```python
from build123d import *

# Parameters (mm, degrees)
SKETCH1_W          = 304.8
SKETCH1_H          = 142.24
EXTRUDE1_DEPTH     = 2.032
SKETCH3_R          = 1.5875
CUT_EXTRUDE1_DEPTH = 252.699806613
SKETCH4_R          = 4.191
SKETCH4_R_2        = 1.5875
SKETCH4_R_3        = 5.842
SKETCH4_W          = 80.01
SKETCH4_H          = 44.958
SKETCH4_W_2        = 29.972
SKETCH4_H_2        = 29.972
EXTRUDE2_DEPTH     = 252.699806613


with BuildPart() as part:
    # Sketch1 → Extrude1 (new body)
    with BuildSketch(Plane.XY):
        with Locations((55.245, 71.12)):
            Rectangle(SKETCH1_W, SKETCH1_H)
    extrude(amount=EXTRUDE1_DEPTH)

    # Sketch3 → Cut-Extrude1 (cut, through all)
    with BuildSketch(Plane.XY.offset(2.032)):
        with Locations((-90.805, 135.89)):
            Circle(SKETCH3_R)
        with Locations((-90.805, 6.35)):
            Circle(SKETCH3_R)
        with Locations((6.35, 135.89)):
            Circle(SKETCH3_R)
        with Locations((6.35, 6.35)):
            Circle(SKETCH3_R)
        with Locations(Location((104.14, 6.35, 0), (0, 0, 180))):
            Circle(SKETCH3_R)
        with Locations(Location((104.14, 135.89, 0), (0, 0, 180))):
            Circle(SKETCH3_R)
        with Locations(Location((201.295, 6.35, 0), (0, 0, 180))):
            Circle(SKETCH3_R)
        with Locations(Location((201.295, 135.89, 0), (0, 0, 180))):
            Circle(SKETCH3_R)
    extrude(amount=-CUT_EXTRUDE1_DEPTH, mode=Mode.SUBTRACT)

    # Sketch4 → Extrude2 (cut, through all)
    with BuildSketch(Plane.XY.offset(2.032)):
        with Locations((38.895, 51.84)):
            Circle(SKETCH4_R)
        with Locations((-43.18, 137.16)):
            Circle(SKETCH4_R_2)
        with Locations((177.165, 104.14)):
            Circle(SKETCH4_R_3)
        with Locations((-21.844, 80.137)):
            Rectangle(SKETCH4_W, SKETCH4_H)
        with Locations((46.609, 79.502)):
            Rectangle(SKETCH4_W_2, SKETCH4_H_2)
    extrude(amount=-EXTRUDE2_DEPTH, mode=Mode.SUBTRACT)


solid = part.part
```
Read the model definition and answer for the solid it produces. Units are mm, in the model's axes. Give positions to 0.01 mm unless a question says otherwise; leave off trailing zeros. Order: outer loops, then holes, each group sorted by start corner. A loop starts at its lowest first (then second) coordinate and runs counter-clockwise, first axis right, second up.
(1) Find section A-A (y = 83). Give the vertices of the cut face in (x, z) (3 decimals).
(2) Straight lines are drawn through the part: L1, parallel to Y at x = -43.18, z = 1.65; L2, parallel to Y at x = -14, z = 1.2; L3, parallel to X at y = 135.5, z = 0.25 (3 decimals). For each, find the intervals that lie inside material, in ascending order.
(3) For a pull along X with two mould halves and no side action, classify faces 1 (the flat face through (53, 56, 0)), 2 (the cylindrical face through (38.349, 55.995, 1.03)) as released by +X, released by -X, zero draft, split by the parting line, or undercut.
(4) Find section B-B (y = 51.84). Give the vertices of the cut face in (x, z) (3 decimals).
(5) Given pin 1 (3.5 mm diameter, centred on x = 201.295, y = 6.35, fed in from -Z), flat-ended and moving along its own axis, determine where the tip first touches the part or whether it passes through.
(6) Find section C-C (z = 1). Give the number of separate pieces and of enclosed holes in the cut face, plus the area to 3 significant figures.
Result sheet:
1. outline: (-97.155, 0) - (-61.849, 0) - (-61.849, 2.032) - (-97.155, 2.032) - close; (18.161, 0) - (31.623, 0) - (31.623, 2.032) - (18.161, 2.032) - close; (61.595, 0) - (207.645, 0) - (207.645, 2.032) - (61.595, 2.032) - close
2. L1: y = 0 to 57.66, 102.62 to 135.57, 138.75 to 142.24
2. L2: y = 0 to 57.66, 102.62 to 142.24
2. L3: x = -97.155 to -92.344, -89.266 to 4.811, 7.889 to 102.601, 105.679 to 199.756, 202.834 to 207.645
3. face 1: zero draft
3. face 2: undercut
4. outline: (-97.155, 0) - (34.704, 0) - (34.704, 2.032) - (-97.155, 2.032) - close; (43.086, 0) - (207.645, 0) - (207.645, 2.032) - (43.086, 2.032) - close
5. pin 1: stops at z = 0
6. separate pieces: 1
6. enclosed holes: 13
6. area: 38,600 mm2
